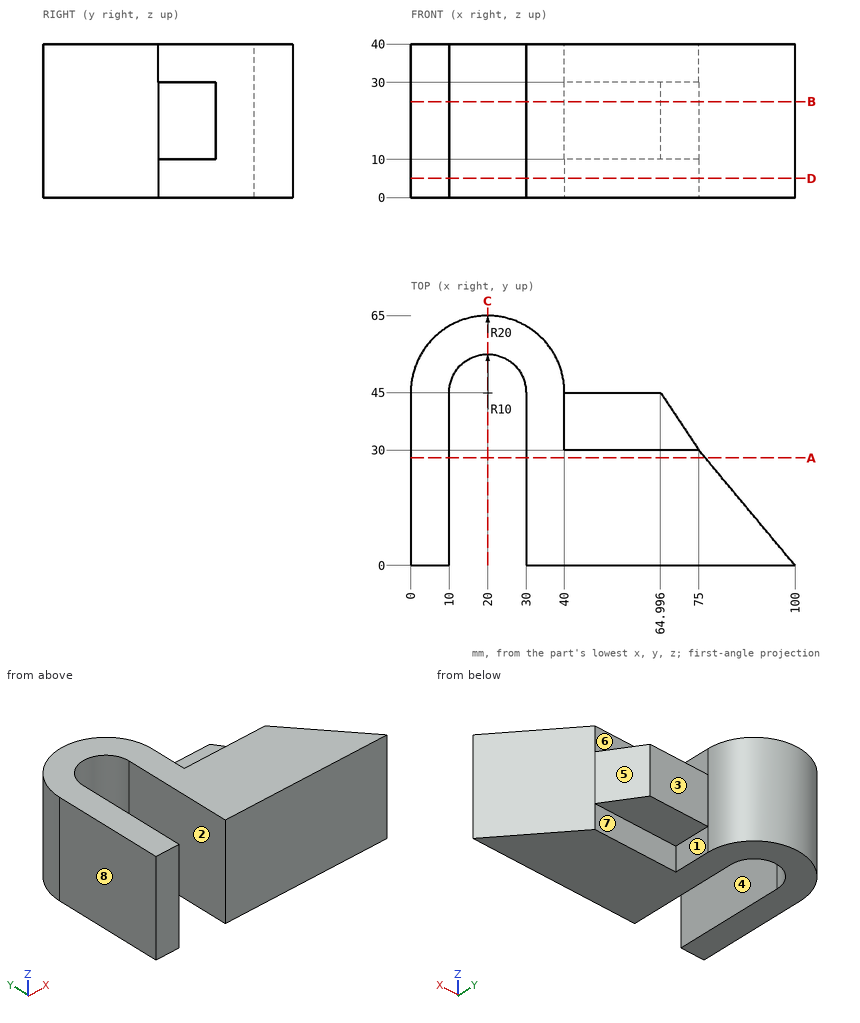
Design review of the part shown in the three views and the two pictorial views. Dimensions are in mm from the part's minimum x, y and z. A direction names the side the tool comes from. Round coordinates to 2 decimals unless told otherwise and drop trailing zeros. Order: outer loops, then holes, each group sorted by start corner. A loop starts at its lowest first (then second) coordinate and runs counter-clockwise, first axis right, second up.
(1) Wall thickness on L1, parallel to Y at x = 72, z = 4.5; L2, parallel to X at y = 51.5, z = 24.5 (1 decimal); L3, parallel to X at y = 3.5, z = 13: over which ranges is each line inside the solid? List them lowest first.
Working result:
L1: y = 0 to 30
L2: x = 1.1 to 12.4, 27.6 to 38.9
L3: x = 0 to 10, 30 to 97.08
(2) For P1, Ø3, axis at x = 55.5, z = 35, coming from the +Y side; P2, Ø10, axis at x = 15.5, y = 47, coming from the +Z side; P3, Ø16.5, axis at x = 51, y = 41, coming from the -Z side; P4, Ø5, axis at y = 38, z = 33.5, coming from the +X side, all flat-tipped, find the tip position at first contact; note any pin that passes through.
Working result:
P1: stops at y = 30
P2: passes through
P3: stops at z = 10
P4: stops at x = 40
(3) Take a section at C-C, the plane x = 20. State the section outline as (y, z) points, plus the area to 3 significant figures.
Working result:
outline: (55, 0) - (65, 0) - (65, 40) - (55, 40) - close
area: 400 mm2
(4) Take a section at D-D, the plane z = 5. State the section outline as (x, y) points, plus the area to 3 significant figures.
Working result:
outline: (0, 0) - (10, 0) - (10, 45) arc R10 cw to (30, 45) - (30, 0) - (100, 0) - (75, 30) - (40, 30) - (40, 45) arc R20 ccw to (0, 45) - close
area: 2,800 mm2
(5) Take a section at A-A, the plane y = 28. State the section outline as (x, z) points.
Working result:
outline: (0, 0) - (10, 0) - (10, 40) - (0, 40) - close; (30, 0) - (76.67, 0) - (76.67, 40) - (30, 40) - close
(6) Mouldability with a two-part tool opening along X and no side actions: class the marked faces 1, 2 and 3 as released by +X, released by -X, zero draft, split by the parting line, or undercut.
Working result:
face 1: released by +X
face 2: undercut
face 3: zero draft
(7) Take a section at B-B, the plane z = 25. State the section outline as (x, y) points.
Working result:
outline: (0, 0) - (10, 0) - (10, 45) arc R10 cw to (30, 45) - (30, 0) - (100, 0) - (75, 30) - (65, 45) - (40, 45) arc R20 ccw to (0, 45) - close
(8) Tool access review of the marked faces 4, 5, 6, 7 and 8: name each direction out of +Z, -Z, +X, -X, +Y, -Y from which nothing blocks a thin tool from reaching the whole face with its end or side.
Working result:
face 4: +Z, -Z, -Y
face 5: +Z, -Z, +X, +Y
face 6: +Z, +X, +Y
face 7: -Z, +X, +Y
face 8: +Z, -Z, -X, +Y, -Y
